Design review of the part built by this model. Coordinates are the model's own, in mm. A direction names the side the tool comes from. Give positions to 0.01 mm unless a question says otherwise; leave off trailing zeros. Loops run counter-clockwise (first coordinate to the right, second up) from the corner with the lowest first, then second, coordinate; pieces in that order, holes last.
from build123d import *

# Parameters (mm, degrees)
SKETCH1_W           = 120
SKETCH1_H           = 140
BOSS_EXTRUDE1_DEPTH = 10
SKETCH2_W           = 74
SKETCH2_H           = 20
BOSS_EXTRUDE2_DEPTH = 5
SKETCH4_R           = 3
SKETCH4_R_2         = 4.5
CUT_EXTRUDE1_DEPTH  = 15


with BuildPart() as part:
    # Sketch1 → Boss-Extrude1 (new body)
    with BuildSketch(Plane.XY):
        with Locations((-60, -70)):
            Rectangle(SKETCH1_W, SKETCH1_H)
    extrude(amount=BOSS_EXTRUDE1_DEPTH)

    # Sketch2 → Boss-Extrude2 (add)
    with BuildSketch(Plane.XY.offset(10)):
        with Locations((-60, -20)):
            Rectangle(SKETCH2_W, SKETCH2_H)
        with Locations((-60, -120)):
            Rectangle(SKETCH2_W, SKETCH2_H)
    extrude(amount=BOSS_EXTRUDE2_DEPTH)

    # Sketch4 → Cut-Extrude1 (cut)
    with BuildSketch(Plane.XY.offset(15)):
        with Locations((-102, -55)):
            Circle(SKETCH4_R)
        with Locations((-60, -55)):
            Circle(SKETCH4_R_2)
        with Locations((-18, -55)):
            Circle(SKETCH4_R)
    extrude(amount=-CUT_EXTRUDE1_DEPTH, mode=Mode.SUBTRACT)


solid = part.part
Q1. Take a section at A-A (x = -102). Give the boundary of the cut face in (y, z).
Results:
outline: (-140, 0) - (-58, 0) - (-58, 10) - (-140, 10) - close; (-52, 0) - (0, 0) - (0, 10) - (-52, 10) - close
Q2. Take a section at B-B (y = -55). Give the boundary of the cut face in (x, z), plus the area to 3 significant figures.
Results:
outline: (-120, 0) - (-105, 0) - (-105, 10) - (-120, 10) - close; (-99, 0) - (-64.5, 0) - (-64.5, 10) - (-99, 10) - close; (-55.5, 0) - (-21, 0) - (-21, 10) - (-55.5, 10) - close; (-15, 0) - (0, 0) - (0, 10) - (-15, 10) - close
area: 990 mm2
Q3. Wall thickness on line 1 (Y direction, x = -55, z = 12.25); line 2 (Z direction, x = -103.5, y = -110); line 3 (Y direction, x = -104, z = 2): over which ranges is each line inside the solid? List them lowest first.
Results:
line 1: y = -130 to -110, -30 to -10
line 2: z = 0 to 10
line 3: y = -140 to -57.24, -52.76 to 0
Q4. Draft analysis for pull direction X (two halves, no side actions). For faces 5 (the face through (-104.21, -52.97, 5.07)), 6 (the face through (-97, -20, 12)), 7 (the face through (-18, -52, 5)), 8 (the face through (-61, -30, 12)), state which applies: pulls with the +X half, pulls with the -X half, needs draft (parallel to the pull), parting line crosses it, or undercut.
Results:
face 5: undercut
face 6: pulls with the -X half
face 7: undercut
face 8: needs draft
Q5. Take a section at C-C (x = -83). Give the boundary of the cut face in (y, z), plus the area to 3 significant figures.
Results:
outline: (-140, 0) - (0, 0) - (0, 10) - (-10, 10) - (-10, 15) - (-30, 15) - (-30, 10) - (-110, 10) - (-110, 15) - (-130, 15) - (-130, 10) - (-140, 10) - close
area: 1,600 mm2
Q6. Insertion check: pin 1 (1.5 mm diameter, centred on y = -17.5, z = 13, fed in from +X); pin 2 (1.5 mm diameter, centred on y = -119.5, z = 13, fed in from -X); pin 3 (1.5 mm diameter, centred on x = -63.5, z = 11.5, fed in from -Y). Each pin has a flat end and moves straight along its axis. Give the tip position at first contact, or say it passes through.
Results:
pin 1: stops at x = -23
pin 2: stops at x = -97
pin 3: stops at y = -130
Q7. Take a section at D-D (x = -60). Give the boundary of the cut face in (y, z), plus the area to 3 significant figures.
Results:
outline: (-140, 0) - (-59.5, 0) - (-59.5, 10) - (-110, 10) - (-110, 15) - (-130, 15) - (-130, 10) - (-140, 10) - close; (-50.5, 0) - (0, 0) - (0, 10) - (-10, 10) - (-10, 15) - (-30, 15) - (-30, 10) - (-50.5, 10) - close
area: 1,510 mm2
Q8. Tool access review of faces 1 (the face through (-23, -20, 12)), 2 (the face through (-61, -130, 12)), 3 (the face through (-61, -10, 12)), 4 (the face through (-61, -110, 12)): name each direction out of +Z, -Z, +X, -X, +Y, -Y from which nothing blocks a thin tool from reaching the whole face with its end or side.
Results:
face 1: +Z, +X, +Y, -Y
face 2: +Z, +X, -X, -Y
face 3: +Z, +X, -X, +Y
face 4: +Z, +X, -X
